Work out the finished part from the listing and answer in its coordinate system (mm). A direction names the side the tool comes from. Coordinates: 2 decimals unless noted, no trailing zeros. Write each loop counter-clockwise with the first axis right and the second up, starting at its lowest first coordinate (ties: lowest second). Pieces come first, ordered by that corner, then holes. Notation, with made-up numbers: (64.25, 48) - (94.25, 48) arc R23 ccw to (94.25, 87) - close; hole circle Ø11 at (24, -11.5). An arc over 180 degrees is marked (long way). Use a Markdown table: item, result. Add a question column.
(1) For a pull along X with two mould halves and no side action, classify faces 4 (the face through (309.75, 30, 0)), 5 (the face through (214.14, 2.46, 76.85)), 6 (the face through (0.04, 2.46, -2.95)) as released by +X, released by -X, zero draft, split by the parting line, or undercut.
(2) A tool of negligible diameter and unlimited length cuts with its end or side. For faces 1 (the face through (101, 60.3, 0)), 2 (the face through (317.992, 2.465, 0.923)), 3 (the face through (194, 5, -9)), from which of +Z, -Z, +X, -X, +Y, -Y can it reach the whole face along a straight path? Write none if from no direction.
(3) The part is cut by section A-A, the plane y = 45. Give the vertices of the cut face in (x, z).
(4) Given pin 1 Ø5.5 at (x, z) = (258.5, 42.5) entering from +Y; pin 2 Ø3 at (y, z) = (10, 35.5) entering from +X; pin 3 Ø1.8 at (y, z) = (11, 35) entering from -X, each flat-ended and moving along its own axis, determine where each tip first touches the part or whether it passes through.
(5) The part is cut by section D-D, the plane z = -203. Give the vertices of the cut face in (x, y), then the cut area to 3 significant figures.
(6) The part is cut by section C-C, the plane x = 263.5. Give the vertices of the cut face in (y, z), then the cut area to 3 significant figures.
(7) Find the intervals of material crossed by line 1 (X direction, y = 49.5, z = -30); line 2 (Z direction, x = 265.5, y = 35.5); line 3 (Y direction, x = 346.5, z = -259), in increasing order. Write a range as from..to.
(8) The part is cut by section B-B, the plane x = 51. Give the vertices of the cut face in (y, z).
from build123d import *

# Parameters (mm, degrees)
EXTRUDE_1_DEPTH          = 5
SKETCH_2_R               = 52
EXTRUDE_2_DEPTH          = 50
SKETCH_3_R               = 7.5
EXTRUDE_3_DEPTH          = 55.3
SKETCH_4_R               = 12.5
EXTRUDE_4_DEPTH          = 3
SKETCH_5_R               = 7.5
EXTRUDE_5_DEPTH          = 11
SKETCH_6_R               = 81.275582603
EXTRUDE_6_DEPTH          = 50
SKETCH_7_R               = 335
EXTRUDE_7_DEPTH          = 5
CUT_EXTRUDE_1_DEPTH      = 632.922060068
CUT_EXTRUDE_1_DEPTH_BACK = 632.922060068
SKETCH_8_W               = 72.819825202
SKETCH_8_H               = 12


with BuildPart() as part:
    # 草图1 → 凸台-拉伸1 (new body)
    with BuildSketch(Plane(origin=(0, 0, 0), x_dir=(1, 0, 0), z_dir=(0, 1, 0))):
        with BuildLine():
            Line((282.724919094, 50.996592885), (147.449838188, 101.993185769))
            ThreePointArc((147.449838188, 101.993185769), (0, 0), (147.449838188, -101.993185769))
            Line((147.449838188, -101.993185769), (282.724919094, -50.996592885))
            ThreePointArc((282.724919094, -50.996592885), (318, 0), (282.724919094, 50.996592885))
        make_face()
    extrude(amount=EXTRUDE_1_DEPTH)

    # 草图2 → 凸台-拉伸2 (add)
    with BuildSketch(Plane(origin=(0, 5, 0), x_dir=(1, 0, 0), z_dir=(0, 1, 0))):
        with Locations(Location((263.5, 0, 0), (0, 0, 270))):
            Circle(SKETCH_2_R)
        with BuildLine():
            Line((217.25, 17.640507362), (217.25, -17.640507362))
            ThreePointArc((217.25, -17.640507362), (263.5, -49.5), (309.75, -17.640507362))
            Line((309.75, -17.640507362), (309.75, 17.640507362))
            ThreePointArc((309.75, 17.640507362), (263.5, 49.5), (217.25, 17.640507362))
        make_face(mode=Mode.SUBTRACT)
    extrude(amount=EXTRUDE_2_DEPTH)

    # 草图3 → 凸台-拉伸3 (add)
    with BuildSketch(Plane(origin=(0, 5, 0), x_dir=(1, 0, 0), z_dir=(0, 1, 0))):
        with Locations(Location((109, 0, 0), (0, 0, 270))):
            Circle(SKETCH_3_R)
    extrude(amount=EXTRUDE_3_DEPTH)

    # 草图4 → 凸台-拉伸4 (add)
    with BuildSketch(Plane(origin=(0, 60.3, 0), x_dir=(1, 0, 0), z_dir=(0, 1, 0))):
        with Locations(Location((109, 0, 0), (0, 0, 270))):
            Circle(SKETCH_4_R)
    extrude(amount=EXTRUDE_4_DEPTH)

    # 草图5 → 凸台-拉伸5 (add)
    with BuildSketch(Plane(origin=(0, 63.3, 0), x_dir=(1, 0, 0), z_dir=(0, 1, 0))):
        with Locations(Location((109, 0, 0), (0, 0, 270))):
            Circle(SKETCH_5_R)
    extrude(amount=EXTRUDE_5_DEPTH)

    # 草图6 → 凸台-拉伸6 (add)
    with BuildSketch(Plane(origin=(0, 5, 0), x_dir=(1, 0, 0), z_dir=(0, 1, 0))):
        with Locations(Location((109, 0, 0), (0, 0, 270))):
            Circle(SKETCH_6_R)
    extrude(amount=EXTRUDE_6_DEPTH)

    # 草图7 → 凸台-拉伸7 (add)
    with BuildSketch(Plane(origin=(0, 0, 0), x_dir=(-1, 0, 0), z_dir=(0, -1, 0))):
        with Locations(Location((-159, 0, 0), (0, 0, 90))):
            Circle(SKETCH_7_R)
    extrude(amount=EXTRUDE_7_DEPTH)

    # 草图8 → 切除-拉伸1 (cut, two sides: drawn at the far end of the back side and taken through both)
    with BuildSketch(Plane.XY.offset(52).offset(-CUT_EXTRUDE_1_DEPTH_BACK)):
        with Locations((263.5, 12)):
            Rectangle(SKETCH_8_W, SKETCH_8_H)
    extrude(amount=CUT_EXTRUDE_1_DEPTH + CUT_EXTRUDE_1_DEPTH_BACK, mode=Mode.SUBTRACT)


solid = part.part
Model answer:
| question | item | result |
|---|---|---|
| 1 | face 4 | undercut |
| 1 | face 5 | released by +X |
| 1 | face 6 | split by the parting line |
| 2 | face 1 | none |
| 2 | face 2 | +X, +Y |
| 2 | face 3 | +Y |
| 3 | outline | circle Ø162.55 at (109, 0); circle Ø104 at (263.5, 0); hole (217.25, -17.64) arc R49.5 ccw to (309.75, -17.64) - (309.75, 17.64) arc R49.5 ccw to (217.25, 17.64) - close |
| 4 | pin 1 | y = 5 |
| 4 | pin 2 | x = 302.84 |
| 4 | pin 3 | x = 35.22 |
| 5 | outline | (-107.49, -5) - (425.49, -5) - (425.49, 0) - (-107.49, 0) - close |
| 5 | area | 2,660 mm^2 |
| 6 | outline | (-5, -318.28) - (0, -318.28) - (0, -58.24) - (5, -58.24) - (5, -52) - (6, -52) - (6, -49.5) - (5, -49.5) - (5, 49.5) - (6, 49.5) - (6, 52) - (5, 52) - (5, 58.24) - (0, 58.24) - (0, 318.28) - (-5, 318.28) - close; (18, -52) - (55, -52) - (55, -49.5) - (18, -49.5) - close; (18, 49.5) - (55, 49.5) - (55, 52) - (18, 52) - close |
| 6 | area | 3,960 mm^2 |
| 7 | line 1 | 33.46..184.54, 221.03..224.13, 302.87..305.97 |
| 7 | line 2 | -51.96..-49.46, 49.46..51.96 |
| 7 | line 3 | -5..0 |
| 8 | outline | (-5, -317.11) - (0, -317.11) - (0, -92.29) - (5, -92.29) - (5, -56.94) - (55, -56.94) - (55, 56.94) - (5, 56.94) - (5, 92.29) - (0, 92.29) - (0, 317.11) - (-5, 317.11) - close |
